Part model, mm, in its own coordinate system. A direction names the side the tool comes from. Give positions to 0.01 mm unless a question says otherwise; leave off trailing zeros. Order: outer loops, then holes, each group sorted by start corner. A loop starts at its lowest first (then second) coordinate and runs counter-clockwise, first axis right, second up. Notation, with made-up numbers: (36, -25) -> (69, -25) arc R13 ccw to (69, -17) -> close; hole circle Ø7 at (6, -40). An arc over 180 degrees is marked (long way). Write item = value, one per line. Start each with the question number.
(1) Flat gauge pins, fed straight in: pin 1 (1.3 mm diameter, centred on x = 8, y = 3, fed in from -Z); pin 2 (1 mm diameter, centred on y = 3.5, z = -1.5, fed in from -X); pin 3 (1 mm diameter, centred on x = -6, y = 2.5, fed in from +Z). Where does each tip first touch, or does it go through?
(2) Saw through at C-C, the plane y = 0.85. List the corners of the cut face in (x, z), then the cut area to 3 significant figures.
(3) Probe line 1 along X through (y, z) = (2.75, 4.75); line 2 along X through (y, z) = (0.8, 2.5); line 3 along Z through (x, y) = (0, 1.8). List the from-to ranges inside material, lowest first. Write a range as from..to.
(4) Saw through at D-D, the plane x = -22.5. List the corners of the cut face in (y, z), then the cut area to 3 significant figures.
(5) Saw through at B-B, the plane z = 4.6. List the corners of the cut face in (x, y).
(6) Two-plate mould, pull along X, no slides. Class faces 1 (the flat face through (22, 2, 7.6)), 2 (the cylindrical face through (-0.54, 2.22, -7.56)), 3 (the flat face through (30.145, 2.218, -12.721)): pulls with the +X half, pulls with the -X half, needs draft (parallel to the pull), parting line crosses it, or undercut.
(7) Which spindle directions (+Z, -Z, +X, -X, +Y, -Y) get a long thin tool onto all of the face, cutting with end or side? Do faces 4 (the flat face through (0, 2, 0)), 5 (the flat face through (27.53, 2.22, -18.59)), 6 (the cylindrical face through (25.74, 2.28, -7.21)). Say none if no direction does.
(8) Saw through at A-A, the plane x = 0. List the corners of the cut face in (y, z), then the cut area to 3 significant figures.
from build123d import *

# Parameters (mm, degrees)
SKETCH1_R           = 1.6
SKETCH1_R_2         = 2.5
BOSS_EXTRUDE1_DEPTH = 4.5
FILLET1_R           = 10
FILLET2_R           = 2.5


with BuildPart() as part:
    # Sketch1 → Boss-Extrude1 (new body)
    with BuildSketch(Plane(origin=(0, 0, 0), x_dir=(1, 0, 0), z_dir=(0, 1, 0))):
        Polygon((-20, 0), (20, 0), (20, -7.6), (25, -7.6), (25, 7.575378798), (34.192388155, 16.767766953), (29.949747468, 21.01040764), (23.939339828, 15), (-23.939339828, 15), (-29.949747468, 21.01040764), (-34.192388155, 16.767766953), (-25, 7.575378798), (-25, -7.6), (-20, -7.6), align=None)
        with Locations((-22.5, -4.6)):
            Circle(SKETCH1_R, mode=Mode.SUBTRACT)
        with Locations((22.5, -4.6)):
            Circle(SKETCH1_R, mode=Mode.SUBTRACT)
        with Locations((-29.949747468, 16.767766953)):
            Circle(SKETCH1_R, mode=Mode.SUBTRACT)
        with Locations((29.949747468, 16.767766953)):
            Circle(SKETCH1_R, mode=Mode.SUBTRACT)
        with Locations((0, 10)):
            Circle(SKETCH1_R_2, mode=Mode.SUBTRACT)
    extrude(amount=BOSS_EXTRUDE1_DEPTH)

    # Fillet1
    fillet1_edges = [part.edges().sort_by_distance(p)[0] for p in [
        (-25, 2.25, -7.575378798),
        (-23.939339828, 2.25, -15),
        (23.939339828, 2.25, -15),
        (25, 2.25, -7.575378798),
    ]]
    fillet(fillet1_edges, radius=FILLET1_R)

    # Fillet2
    fillet2_edges = [part.edges().sort_by_distance(p)[0] for p in [
        (-34.192388155, 2.25, -16.767766953),
        (-29.949747468, 2.25, -21.01040764),
        (29.949747468, 2.25, -21.01040764),
        (34.192388155, 2.25, -16.767766953),
    ]]
    fillet(fillet2_edges, radius=FILLET2_R)


solid = part.part
Results list:
q1.pin_1 = -15
q1.pin_2 = -25
q1.pin_3 = 0
q2.outline = (-32.42, -18.54) -> (-31.72, -19.24) arc R2.5 ccw to (-28.18, -19.24) -> (-26.87, -17.93) arc R10 cw to (-19.8, -15) -> (19.8, -15) arc R10 cw to (26.87, -17.93) -> (28.18, -19.24) arc R2.5 ccw to (31.72, -19.24) -> (32.42, -18.54) arc R2.5 ccw to (32.42, -15) -> (27.93, -10.5) arc R10 cw to (25, -3.43) -> (25, 7.6) -> (20, 7.6) -> (20, 0) -> (-20, 0) -> (-20, 7.6) -> (-25, 7.6) -> (-25, -3.43) arc R10 cw to (-27.93, -10.5) -> (-32.42, -15) arc R2.5 ccw to start; hole circle Ø3.2 at (-29.95, -16.77); hole circle Ø3.2 at (-22.5, 4.6); hole circle Ø5 at (0, -10); hole circle Ø3.2 at (22.5, 4.6); hole circle Ø3.2 at (29.95, -16.77)
q2.area = 899 mm^2
q3.line_1 = -25..-24.09, -20.91..-20, 20..20.91, 24.09..25
q3.line_2 = -25..-20, 20..25
q3.line_3 = -15..-12.5, -7.5..0
q4.outline = (0, -15.37) -> (4.5, -15.37) -> (4.5, 3) -> (0, 3) -> close; (0, 6.2) -> (4.5, 6.2) -> (4.5, 7.6) -> (0, 7.6) -> close
q4.area = 89.0 mm^2
q5.outline = (-25, 0) -> (-24.1, 0) -> (-24.1, 4.5) -> (-25, 4.5) -> close; (-20.9, 0) -> (-20, 0) -> (-20, 4.5) -> (-20.9, 4.5) -> close; (20, 0) -> (20.9, 0) -> (20.9, 4.5) -> (20, 4.5) -> close; (24.1, 0) -> (25, 0) -> (25, 4.5) -> (24.1, 4.5) -> close
q6.face_1 = needs draft
q6.face_2 = undercut
q6.face_3 = pulls with the +X half
q7.face_4 = +Z, +Y, -Y
q7.face_5 = -Z, +Y, -Y
q7.face_6 = +Z, +X, +Y, -Y
q8.outline = (0, -15) -> (4.5, -15) -> (4.5, -12.5) -> (0, -12.5) -> close; (0, -7.5) -> (4.5, -7.5) -> (4.5, 0) -> (0, 0) -> close
q8.area = 45.0 mm^2
